```python
from build123d import *

# Parameters (mm, degrees)
SKETCH_R          = 4.25
PAD_DEPTH         = 28.5
PAD_DEPTH_BACK    = 5
FILLET_R          = 5
SKETCH002_R       = 6.4
POCKET_DEPTH      = 24.001
POCKET_DEPTH_BACK = -16.001
POCKET001_DEPTH   = 3
POCKET002_DEPTH   = 4
POCKET003_DEPTH   = 101.201
POCKET004_DEPTH   = 4
POCKET005_DEPTH   = 16
SKETCH028_R       = 22
POCKET006_DEPTH   = 25
SKETCH031_R       = 2.2
POCKET007_DEPTH   = 9
PAD001_DEPTH      = 17.2
SKETCH038_W       = 50
SKETCH038_H       = 26
POCKET008_DEPTH   = 2
SKETCH039_R       = 4.4
POCKET009_DEPTH   = 1.5
CHAMFER_SIZE      = 1.8
CHAMFER001_SIZE   = 2.8


with BuildPart() as part:
    # Sketch → Pad (new body, two sides)
    with BuildSketch(Plane.XY) as pad_sk:
        with BuildLine():
            ThreePointArc((0, -19), (16, -3), (0, 13))
            Line((0, 44.1), (0, 13))
            ThreePointArc((0, 44.1), (-2.928932, 51.171068), (-10, 54.1))
            Line((-24, 54.1), (-10, 54.1))
            Line((-24, 54.1), (-24, -47.1))
            Line((-24, -47.1), (-1, -47.1))
            ThreePointArc((-1, -47.1), (-0.292893, -46.807107), (0, -46.1))
            Line((0, -19), (0, -46.1))
        make_face()
        with Locations((0, -3)):
            Circle(SKETCH_R, mode=Mode.SUBTRACT)
    extrude(amount=PAD_DEPTH)
    extrude(pad_sk.sketch, amount=-PAD_DEPTH_BACK)

    # Fillet
    fillet_edges = [part.edges().sort_by_distance(p)[0] for p in [
        (0, 13, 11.75),
        (0, -19, 11.75),
    ]]
    fillet(fillet_edges, radius=FILLET_R)

    # Sketch002 → Pocket (cut, two sides)
    with BuildSketch(Plane.YZ) as pocket_sk:
        with Locations((-30, 11.5)):
            Circle(SKETCH002_R)
        with Locations((40, 11.5)):
            Circle(SKETCH002_R)
    extrude(amount=-POCKET_DEPTH, mode=Mode.SUBTRACT)
    extrude(pocket_sk.sketch, amount=-POCKET_DEPTH_BACK, mode=Mode.SUBTRACT)

    # Sketch013 → Pocket001 (cut)
    with BuildSketch(Plane.XY.offset(28.5)):
        with BuildLine():
            ThreePointArc((0, -13), (10, -3), (0, 7))
            Line((-40, 7), (0, 7))
            Line((-40, 7), (-40, 60))
            Line((-40, 60), (30, 60))
            Line((30, 60), (30, -60))
            Line((30, -60), (-40, -60))
            Line((-40, -60), (-40, -13))
            Line((-40, -13), (0, -13))
        make_face()
    extrude(amount=-POCKET001_DEPTH, mode=Mode.SUBTRACT)

    # Sketch024 → Pocket002 (cut)
    with BuildSketch(Plane(origin=(0, 0, -5), x_dir=(1, 0, 0), z_dir=(0, 0, -1))):
        with BuildLine():
            Line((0, 13), (-40, 13))
            Line((-40, 13), (-40, 65))
            Line((-40, 65), (24, 65))
            Line((24, 65), (24, -65))
            Line((24, -65), (-40, -65))
            Line((-40, -7), (-40, -65))
            Line((-40, -7), (0, -7))
            ThreePointArc((0, -7), (10, 3), (0, 13))
        make_face()
    extrude(amount=-POCKET002_DEPTH, mode=Mode.SUBTRACT)

    # Sketch029 → Pocket003 (cut, through all)
    with BuildSketch(Plane(origin=(0, 54.1, 0), x_dir=(-1, 0, 0), z_dir=(0, 1, 0))):
        with BuildLine():
            ThreePointArc((32, 30), (13.221825, 37.778175), (21, 19))
            Line((21, 19), (32, 19))
            Line((32, 30), (32, 19))
        make_face()
    extrude(amount=-POCKET003_DEPTH, mode=Mode.SUBTRACT)

    # Sketch027 → Pocket004 (cut)
    with BuildSketch(Plane(origin=(0, 0, -5), x_dir=(1, 0, 0), z_dir=(0, 0, -1))):
        Polygon((3.925982, 9.8), (-3.925982, 9.8), (-7.851964, 3), (-3.925982, -3.8), (3.925982, -3.8), (7.851964, 3), align=None)
    extrude(amount=-POCKET004_DEPTH, mode=Mode.SUBTRACT)

    # Sketch025 → Pocket005 (cut, symmetric)
    with BuildSketch(Plane.YZ):
        with BuildLine():
            Line((-16, 20.1), (26, 20.1))
            ThreePointArc((30, 16), (28.864001, 18.892928), (26, 20.1))
            Line((30, 16), (30, 7))
            ThreePointArc((26, 2.9), (28.864001, 4.107072), (30, 7))
            Line((26, 2.9), (-16, 2.9))
            ThreePointArc((-20, 7), (-18.864001, 4.107072), (-16, 2.9))
            Line((-20, 7), (-20, 16))
            ThreePointArc((-16, 20.1), (-18.864001, 18.892928), (-20, 16))
        make_face()
    extrude(amount=POCKET005_DEPTH, both=True, mode=Mode.SUBTRACT)

    # Sketch028 → Pocket006 (cut)
    with BuildSketch(Plane(origin=(0, 54.1, 0), x_dir=(-1, 0, 0), z_dir=(0, 1, 0))):
        with Locations((21, -20)):
            Circle(SKETCH028_R)
    extrude(amount=-POCKET006_DEPTH, mode=Mode.SUBTRACT)

    # Sketch031 → Pocket007 (cut)
    with BuildSketch(Plane(origin=(0, 0, -1), x_dir=(1, 0, 0), z_dir=(0, 0, -1))):
        with Locations((-6, 30)):
            Circle(SKETCH031_R)
        with Locations((-6, -40)):
            Circle(SKETCH031_R)
    extrude(amount=-POCKET007_DEPTH, mode=Mode.SUBTRACT)

    # Sketch032 → Pad001 (new body)
    with BuildSketch(Plane.XY.offset(2.9)):
        Polygon((0, -22), (-16, -11.5), (-16, -22), align=None)
        Polygon((-16, 12), (0, 30.1), (-16, 30.1), align=None)
    extrude(amount=PAD001_DEPTH)

    # Sketch038 → Pocket008 (cut)
    with BuildSketch(Plane(origin=(0, 0, -5), x_dir=(1, 0, 0), z_dir=(0, 0, -1))):
        with Locations((-10, 2)):
            Rectangle(SKETCH038_W, SKETCH038_H)
    extrude(amount=-POCKET008_DEPTH, mode=Mode.SUBTRACT)

    # Sketch039 → Pocket009 (cut)
    with BuildSketch(Plane(origin=(0, 0, -1), x_dir=(1, 0, 0), z_dir=(0, 0, -1))):
        with Locations((-6, 30)):
            Circle(SKETCH039_R)
        with Locations((-6, -40)):
            Circle(SKETCH039_R)
    extrude(amount=-POCKET009_DEPTH, mode=Mode.SUBTRACT)

    # Chamfer
    chamfer_edges = [part.edges().sort_by_distance(p)[0] for p in [
        (-12, -13, -1),
        (10, -3, -1),
        (-12, 7, -1),
    ]]
    chamfer(chamfer_edges, length=CHAMFER_SIZE)

    # Chamfer001
    chamfer001_edges = [part.edges().sort_by_distance(p)[0] for p in [
        (-5.481285, 7, 25.5),
        (10, -3, 25.5),
        (-5.481285, -13, 25.5),
    ]]
    chamfer(chamfer001_edges, length=CHAMFER001_SIZE)


solid = part.part
```
Check sheet for the modelled part. Datum: model origin and axes. Units: mm. A direction names the side the tool comes from. Round coordinates to 2 decimals unless told otherwise and drop trailing zeros. Order: outer loops, then holes, each group sorted by start corner. A loop starts at its lowest first (then second) coordinate and runs counter-clockwise, first axis right, second up. Notation, with made-up numbers: (24.25, 71) -> (48.25, 71) arc R26 ccw to (48.25, 110) -> close; hole circle Ø4 at (46.5, 67). An arc over 180 degrees is marked (long way). One line per item, written item: value. Start each with the question number.
Q1. Mould release check, pull along X, two halves, no side actions. Record for faces 1 (the face through (-16, 0, 12)), 2 (the face through (-8.198, -30.097, 2.96)), 3 (the face through (-3.3, 0, 20.1)): pulls with the +X half, pulls with the -X half, needs draft (parallel to the pull), parting line crosses it, or undercut.
Q2. Cross-section at A-A (y = -30). Record the boundary of the cut face in (x, z).
Q3. Gauge pin test, flat ends, axial feed: pin 1 Ø10 at (x, y) = (0, -3) entering from -Z; pin 2 Ø9.5 at (x, y) = (3, 13) entering from +Z; pin 3 Ø10 at (y, z) = (-17, 21.5) entering from -X; pin 4 Ø2.5 at (x, y) = (-6, -30) entering from -Z. Record the tip position at first contact, or that the pin passes through.
Q4. Set-up check for faces 4 (the face through (0, 31, 12)), 5 (the face through (0, -37, 12)), 6 (the face through (5.86, 0.45, -2.01)), 7 (the face through (-11, -3, -3)), 8 (the face through (-0.98, 27.68, 3.27)): record each of +Z, -Z, +X, -X, +Y, -Y from which the full face is reachable in a straight line by a thin tool's end or side.
Q5. Thickness scan on line 1 (X direction, y = -30, z = 3); line 2 (Z direction, x = 14, y = -4); line 3 (X direction, y = -30, z = -0.2). Record the ranges inside material, lowest first.
Q6. Cross-section at C-C (x = -20). Record the boundary of the cut face in (y, z), and give its area (3 significant figures).
Q7. Cross-section at B-B (z = 11.5). Record the boundary of the cut face in (x, y).
Q8. Cross-section at D-D (y = 14). Record the boundary of the cut face in (x, z).
Completed:
1. face 1: pulls with the +X half
1. face 2: undercut
1. face 3: needs draft
2. outline: (-24, -1) -> (-10.4, -1) -> (-10.4, 0.5) -> (-8.2, 0.5) -> (-8.2, 5.1) -> (-24, 5.1) -> close; (-24, 17.9) -> (0, 17.9) -> (0, 25.5) -> (-10.96, 25.5) arc R11 cw to (-21, 19) -> (-24, 19) -> close; (-3.8, 0.5) -> (-1.6, 0.5) -> (-1.6, -1) -> (0, -1) -> (0, 5.1) -> (-3.8, 5.1) -> close
3. pin 1: stops at z = -1
3. pin 2: stops at z = 26.77
3. pin 3: stops at x = -24
3. pin 4: stops at z = 17.78
4. face 4: +Z, -Z, +X, +Y
4. face 5: +Z, -Z, +X, -Y
4. face 6: -Z
4. face 7: -Z, +X, -X, +Y, -Y
4. face 8: +X
5. line 1: x = -24 to -8.2, -3.8 to 0
5. line 2: z = -1 to 2.9, 20.1 to 25.5
5. line 3: x = -24 to -10.4, -1.6 to 0
6. outline: (-47.1, -1) -> (-14.8, -1) -> (-13, -2.8) -> (-13, -3) -> (7, -3) -> (7, -2.8) -> (8.8, -1) -> (29.1, -1) -> (29.1, 1.98) -> (54.1, 1.98) -> (54.1, 19.05) -> (-47.1, 19.05) -> close; hole circle Ø12.8 at (-30, 11.5); hole circle Ø12.8 at (40, 11.5)
6. area: 1,740 mm²
7. outline: (-24, -47.1) -> (-1, -47.1) arc R1 ccw to (0, -46.1) -> (0, -36.4) -> (-24, -36.4) -> close; (-24, -23.6) -> (0, -23.6) -> (0, -23.4) arc R5 cw to (1.33, -20) -> (-3.05, -20) -> (-16, -11.5) -> (-16, 12) -> (-0.09, 30) -> (0, 30) -> (0, 33.6) -> (-24, 33.6) -> close; (-24, 46.4) -> (-0.27, 46.4) arc R10 ccw to (-10, 54.1) -> (-24, 54.1) -> close
8. outline: (-24, -1) -> (1.33, -1) -> (1.33, 2.9) -> (-14.23, 2.9) -> (-14.23, 20.1) -> (1.33, 20.1) -> (1.33, 25.5) -> (-10.96, 25.5) arc R11 cw to (-21, 19) -> (-24, 19) -> close
